from build123d import *

# Parameters (mm, degrees)
F2_DEPTH = 6.5
F3_R     = 1
F4_R     = 0.3


with BuildPart() as f2:
    # F1 (on Right) → F2 (new body, symmetric)
    with BuildSketch(Plane.YZ):
        Polygon((59.5, 0), (0, 0), (0, 7), (-1, 7), (-1, 17), (1.5, 27), (-3, 27), (-3, -3), (0, -3), (59.5, -3), (62.5, -3), (62.5, 4.1), (59.75, 6.85), (57, 4.1), (57, 1.85), (59.5, 1.85), align=None)
    extrude(amount=F2_DEPTH, both=True)

    # F3
    f3_edges = [f2.edges().sort_by_distance(p)[0] for p in [
        (0, 62.5, -3),
        (0, -3, -3),
        (0, -3, 27),
        (0, 62.5, 4.1),
        (0, 59.75, 6.85),
        (0, 57, 4.1),
        (0, 0, 0),
    ]]
    fillet(f3_edges, radius=F3_R)

    # F4
    f4_edges = [f2.edges().sort_by_distance(p)[0] for p in [
        (0, -1, 17),
        (0, 59.5, 0),
        (0, 59.5, 1.85),
        (0, 0, 7),
        (0, -1, 7),
    ]]
    fillet(f4_edges, radius=F4_R)


solid = f2.part
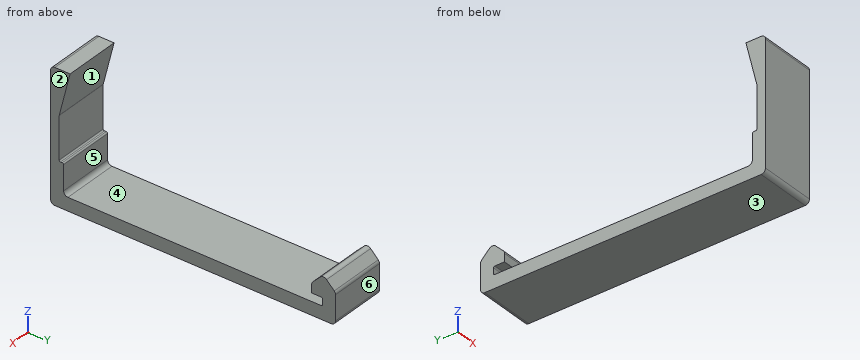
Source: CAD feature listing. Evaluate the final solid. Frame: model axes, mm. Face numbers are marked on the shaded views. A direction names the side the tool comes from. Round coordinates to 2 decimals unless told otherwise and drop trailing zeros. Loops run counter-clockwise (first coordinate to the right, second up) from the corner with the lowest first, then second, coordinate; pieces in that order, holes last. Notation, with made-up numbers: (82.5, 61) -> (100.5, 61) arc R15 ccw to (100.5, 67) -> close; hole circle Ø7 at (23.25, 79). An arc over 180 degrees is marked (long way). Answer as a JSON object with one key per item and string values. Group by question number.
Q1. Ray query, line 1 (Y direction, x = -3.25, z = 3.75); line 2 (Y direction, x = -4, z = 25); line 3 (Z direction, x = 1.5, y = 5). Return the intervals inside material, ascending. Write a range as from..to.
Q2. Contact query for flat-ended pins moving along their axis: P1, Ø5, axis at x = 1, y = 11.5, coming from the +Z side; P2, Ø5, axis at x = 3, z = 14.5, coming from the +Y side. Output: stop coordinate, or through.
Q3. Access query for the marked faces 1 and 2. Directions: +Z, -Z, +X, -X, +Y, -Y. A direction counts if a zero-diameter tool reaches every point of the face in a straight line with its end or side. Return the directions, or none.
Q4. Section query A-A (z = 3). Output: boundary loops of the cut face in (x, y).
Q5. Mould query, pull axis Y, two halves, no side actions, for the marked faces 3, 4, 5 and 6. Classes: pulls with the +Y half, pulls with the -Y half, needs draft (parallel to the pull), parting line crosses it, or undercut.
Q6. Section query D-D (y = 24). Output: boundary loops of the cut face in (x, z).
Q7. Section query B-B (x = 2.5). Output: boundary loops of the cut face in (y, z).
Q8. Section query C-C (z = 25). Output: boundary loops of the cut face in (x, y), plus the area to 3 significant figures.
Completed:
{
 "1": {"line 1": "-3..0, 57..62.5", "line 2": "-3..1", "line 3": "-3..0"},
 "2": {"P1": "z = 0", "P2": "y = -1"},
 "3": {"face 1": "+X, -X, +Y", "face 2": "+Z, -Z, +X, +Y, -Y"},
 "4": {"outline": "(-6.5, -3) -> (6.5, -3) -> (6.5, 0) -> (-6.5, 0) -> close; (-6.5, 57) -> (6.5, 57) -> (6.5, 62.5) -> (-6.5, 62.5) -> close"},
 "5": {"face 3": "needs draft", "face 4": "undercut", "face 5": "undercut", "face 6": "pulls with the +Y half"},
 "6": {"outline": "(-6.5, -3) -> (6.5, -3) -> (6.5, 0) -> (-6.5, 0) -> close"},
 "7": {"outline": "(-3, -2) arc R1 ccw to (-2, -3) -> (61.5, -3) arc R1 ccw to (62.5, -2) -> (62.5, 3.69) arc R1 ccw to (62.21, 4.39) -> (60.46, 6.14) arc R1 ccw to (59.04, 6.14) -> (57.29, 4.39) arc R1 ccw to (57, 3.69) -> (57, 1.85) -> (59.2, 1.85) arc R0.3 cw to (59.5, 1.55) -> (59.5, 0.3) arc R0.3 cw to (59.2, 0) -> (1, 0) arc R1 cw to (0, 1) -> (0, 6.7) arc R0.3 ccw to (-0.3, 7) -> (-0.7, 7) arc R0.3 cw to (-1, 7.3) -> (-1, 16.96) arc R0.3 cw to (-0.99, 17.04) -> (1.5, 27) -> (-2, 27) arc R1 ccw to (-3, 26) -> close"},
 "8": {"outline": "(-6.5, -3) -> (6.5, -3) -> (6.5, 1) -> (-6.5, 1) -> close", "area": "52.0 mm²"}
}
